The listing builds one solid part. Answer for the finished solid, in the listing's coordinates (mm). A direction names the side the tool comes from. Round coordinates to 2 decimals unless told otherwise and drop trailing zeros. Loops run counter-clockwise (first coordinate to the right, second up) from the corner with the lowest first, then second, coordinate; pieces in that order, holes last. Notation, with made-up numbers: M 37,65 L 54,65 A35 cw 54,97 Z; hole C -27,52.25 d11. An arc over 180 degrees is marked long. Put each result on its own line as item: value. Start each with the question number.
(1) Section A-A, the plane z = -57 is taken. Determine the outline of the cut face in (x, y), then the cut area to 3 significant figures.
(2) Straight lines are drawn through the part: line 1 (X direction, y = 3.7, z = 67); line 2 (X direction, y = 1.7, z = -13); line 3 (Z direction, x = -5, y = 2.45). For each, find the intervals that lie inside material, in ascending order.
(3) Which of the six approach directions +Z, -Z, +X, -X, +Y, -Y give full straight-line access (tool end or side, diameter ignored) to faces 1 (the face through (-53, 2, 54.338)), 2 (the face through (-30, 2, 5)), 3 (the face through (52, 2, 54.338))?
(4) Determine the mould class of faces 4 (the face through (-1, 2, 75)), 5 (the face through (50, 2, 61)), 6 (the face through (30, 2, 15)) for opening direction X: released by +X, released by -X, zero draft, split by the parting line, or undercut.
(5) Section B-B, the plane y = 2.6 is taken. Count the separate pieces of the cut face and the enclosed holes in it, then the cut area to 3 significant figures.
(6) Flat-ended cylindrical pins translate along their axes: P1, Ø0.7, axis at x = -52.5, y = 1.5, coming from the -Z side; P2, Ø2, axis at y = 4, z = 21.5, coming from the +X side; P3, Ø1.5, axis at x = 53, y = 2, coming from the +Z side. Find the tip coordinate at first contact, or state that the pin passes through.
```python
from build123d import *

# Parameters (mm, degrees)
SKETCH1_R           = 1.6
SKETCH1_W           = 10
SKETCH1_H           = 10
SKETCH1_R_2         = 1.5
SKETCH1_W_2         = 35
SKETCH1_H_2         = 4
BOSS_EXTRUDE1_DEPTH = 5
FILLET1_R           = 10
FILLET2_R           = 2
FILLET3_R           = 3
FILLET4_R           = 1
FILLET5_R           = 1


# Some blends are built 0.0001 mm under size
with BuildPart() as part:
    # Sketch1 → Boss-Extrude1 (new body)
    with BuildSketch(Plane(origin=(0, 0, 0), x_dir=(1, 0, 0), z_dir=(0, 1, 0))):
        Polygon((55, 75), (-55, 75), (-55, -18.337824516), (-50, -18.337824516), (-50, -32.337824516), (-55, -32.337824516), (-55, -54.337824516), (-50, -54.337824516), (-50, -68.337824516), (-55, -68.337824516), (-55, -75), (55, -75), (55, -68.337824516), (50, -68.337824516), (50, -54.337824516), (55, -54.337824516), (55, -32.337824516), (50, -32.337824516), (50, -18.337824516), (55, -18.337824516), align=None)
        with Locations(Location((-45.3, -29.437824516, 0), (0, 0, 270))):
            Circle(SKETCH1_R, mode=Mode.SUBTRACT)
        with Locations((-30, -10)):
            Rectangle(SKETCH1_W, SKETCH1_H, mode=Mode.SUBTRACT)
        with Locations(Location((-17.5, -5, 0), (0, 0, 270))):
            Circle(SKETCH1_R_2, mode=Mode.SUBTRACT)
        with Locations(Location((17.5, -5, 0), (0, 0, 270))):
            Circle(SKETCH1_R_2, mode=Mode.SUBTRACT)
        with Locations(Location((45.3, -29.437824516, 0), (0, 0, 270))):
            Circle(SKETCH1_R, mode=Mode.SUBTRACT)
        with Locations((30, -10)):
            Rectangle(SKETCH1_W, SKETCH1_H, mode=Mode.SUBTRACT)
        with Locations(Location((-40, 13, 0), (0, 0, 270))):
            Circle(SKETCH1_R_2, mode=Mode.SUBTRACT)
        with Locations((0, 30)):
            Rectangle(SKETCH1_W_2, SKETCH1_H_2, mode=Mode.SUBTRACT)
        with Locations(Location((-30.5, 62, 0), (0, 0, 270))):
            Circle(SKETCH1_R_2, mode=Mode.SUBTRACT)
        with Locations(Location((-18.65, 57, 0), (0, 0, 270))):
            Circle(SKETCH1_R_2, mode=Mode.SUBTRACT)
        with Locations(Location((-15, 69.897229132, 0), (0, 0, 270))):
            Circle(SKETCH1_R_2, mode=Mode.SUBTRACT)
        with Locations(Location((40, 13, 0), (0, 0, 270))):
            Circle(SKETCH1_R_2, mode=Mode.SUBTRACT)
        with Locations(Location((18.65, 57, 0), (0, 0, 270))):
            Circle(SKETCH1_R_2, mode=Mode.SUBTRACT)
        with Locations(Location((15, 69.897229132, 0), (0, 0, 270))):
            Circle(SKETCH1_R_2, mode=Mode.SUBTRACT)
        with Locations(Location((30.5, 62, 0), (0, 0, 270))):
            Circle(SKETCH1_R_2, mode=Mode.SUBTRACT)
        with Locations(Location((-45.3, -57.237824516, 0), (0, 0, 270))):
            Circle(SKETCH1_R, mode=Mode.SUBTRACT)
        with Locations(Location((-40, -67, 0), (0, 0, 270))):
            Circle(SKETCH1_R_2, mode=Mode.SUBTRACT)
        with Locations(Location((-17.5, -55, 0), (0, 0, 270))):
            Circle(SKETCH1_R_2, mode=Mode.SUBTRACT)
        with Locations(Location((17.5, -55, 0), (0, 0, 270))):
            Circle(SKETCH1_R_2, mode=Mode.SUBTRACT)
        with Locations(Location((40, -67, 0), (0, 0, 270))):
            Circle(SKETCH1_R_2, mode=Mode.SUBTRACT)
        with Locations(Location((45.3, -57.237824516, 0), (0, 0, 270))):
            Circle(SKETCH1_R, mode=Mode.SUBTRACT)
    extrude(amount=BOSS_EXTRUDE1_DEPTH)

    # Fillet1
    # the kernel refuses this fillet: 10 mm, written as the material it takes off along each edge
    with BuildSketch(Plane(origin=(55, -23.566253348, 75), x_dir=(-1, 0, 0), z_dir=(0, 1, 0))) as fillet1_piece_1:
        with BuildLine():
            CenterArc((9.426501339, -10), FILLET1_R, 90, 70.501483543)
            Line((0, -6.662175484), (-0.188530027, -6.595418994))
            ThreePointArc((-0.188530027, -6.595418994), (-0.2, -3.331087742), (-0.2, 0))
            Line((-0.2, 0), (0, 0.2))
            Line((0, 0.2), (9.426501339, 0.2))
            Line((9.426501339, 0.2), (9.426501339, 0))
        make_face()
    extrude(amount=52.132506697, mode=Mode.SUBTRACT)
    with BuildSketch(Plane(origin=(-55, -23.566253348, 75), x_dir=(0, 0, -1), z_dir=(0, 1, 0))) as fillet1_piece_2:
        with BuildLine():
            CenterArc((10, -9.426501339), FILLET1_R, 109.498516457, 70.501483543)
            Line((0, -9.426501339), (-0.2, -9.426501339))
            Line((-0.2, -9.426501339), (-0.2, 0))
            Line((-0.2, 0), (0, 0.2))
            ThreePointArc((0, 0.2), (3.331087742, 0.2), (6.595418994, 0.188530027))
            Line((6.595418994, 0.188530027), (6.662175484, 0))
        make_face()
    extrude(amount=52.132506697, mode=Mode.SUBTRACT)
    with BuildSketch(Plane(origin=(-55, -25, -75), x_dir=(1, 0, 0), z_dir=(0, 1, 0)), Plane(origin=(55, -25, -75), x_dir=(0, 0, 1), z_dir=(0, 1, 0))) as fillet1_piece_3:
        with BuildLine():
            CenterArc((FILLET1_R, -FILLET1_R), FILLET1_R, 90, 90)
            Line((0, -FILLET1_R), (-FILLET1_R * 0.02, -FILLET1_R))
            Line((-FILLET1_R * 0.02, -FILLET1_R), (-FILLET1_R * 0.02, FILLET1_R * 0.02))
            Line((-FILLET1_R * 0.02, FILLET1_R * 0.02), (FILLET1_R, FILLET1_R * 0.02))
            Line((FILLET1_R, FILLET1_R * 0.02), (FILLET1_R, 0))
        make_face()
    extrude(amount=55, mode=Mode.SUBTRACT)

    # Fillet2
    fillet2_edges = [part.edges().sort_by_distance(p)[0] for p in [
        (-17.5, 2.5, -28),
        (-17.5, 2.5, -32),
        (17.5, 2.5, -28),
        (17.5, 2.5, -32),
    ]]
    fillet(fillet2_edges, radius=FILLET2_R - 0.0001)  # a hair under: the kernel refuses the full size

    # Fillet3
    fillet3_edges = [part.edges().sort_by_distance(p)[0] for p in [
        (25, 2.5, 5),
        (25, 2.5, 15),
        (35, 2.5, 15),
        (35, 2.5, 5),
        (-35, 2.5, 5),
        (-35, 2.5, 15),
        (-25, 2.5, 15),
        (-25, 2.5, 5),
    ]]
    fillet(fillet3_edges, radius=FILLET3_R)

    # Fillet4
    fillet4_edges = [part.edges().sort_by_distance(p)[0] for p in [
        (-55, 2.5, 68.337824516),
        (-50, 2.5, 68.337824516),
        (-50, 2.5, 54.337824516),
        (-55, 2.5, 54.337824516),
        (-55, 2.5, 32.337824516),
        (-50, 2.5, 32.337824516),
        (-50, 2.5, 18.337824516),
        (-55, 2.5, 18.337824516),
    ]]
    fillet(fillet4_edges, radius=FILLET4_R)

    # Fillet5
    fillet5_edges = [part.edges().sort_by_distance(p)[0] for p in [
        (55, 2.5, 54.337824516),
        (50, 2.5, 54.337824516),
        (50, 2.5, 68.337824516),
        (55, 2.5, 68.337824516),
        (55, 2.5, 18.337824516),
        (50, 2.5, 18.337824516),
        (50, 2.5, 32.337824516),
        (55, 2.5, 32.337824516),
    ]]
    fillet(fillet5_edges, radius=FILLET5_R)


solid = part.part
```
Recorded:
1. outline: M -55,0 L -20.15,0 L -20.15,5 L -55,5 Z; M -17.15,0 L 17.15,0 L 17.15,5 L -17.15,5 Z; M 20.15,0 L 55,0 L 55,5 L 20.15,5 Z
1. area: 520 mm²
2. line 1: x = -50 to -41.5, -38.5 to 38.5, 41.5 to 50
2. line 2: x = -55 to -41.5, -38.5 to 38.5, 41.5 to 55
2. line 3: z = -75 to -32, -28 to 75
3. face 1: -X, +Y, -Y
3. face 2: +Y, -Y
3. face 3: +X, +Y, -Y
4. face 4: zero draft
4. face 5: released by +X
4. face 6: undercut
5. separate pieces: 1
5. enclosed holes: 21
5. area: 15,700 mm²
6. P1: stops at z = -71.99
6. P2: stops at x = 50
6. P3: stops at z = 72.44
